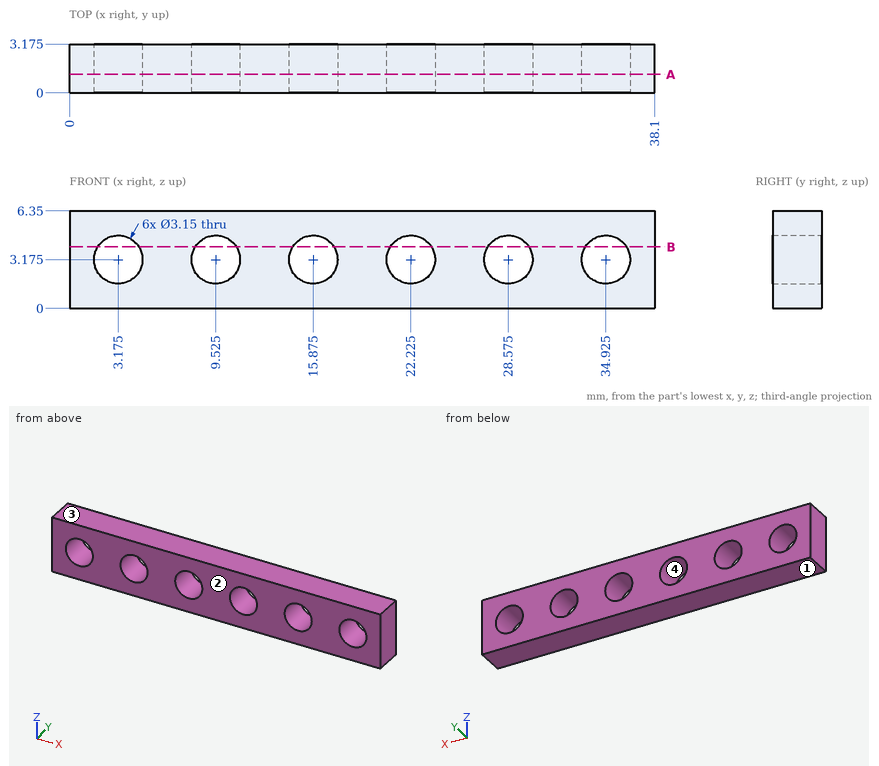
The drawing under review shows one solid part. Ordinate dimensions are in mm from its lowest x, y, z. Round coordinates to 2 decimals unless told otherwise and drop trailing zeros. Write each loop counter-clockwise with the first axis right and the second up, starting at its lowest first coordinate (ties: lowest second). Pieces come first, ordered by that corner, then holes.
(1) Wall thickness on L1, parallel to Z at x = 35, y = 0.95; L2, parallel to Z at x = 2.5, y = 2.3: over which ranges is each line inside the solid? List them lowest first.
(2) We need section A-A on y = 1.2. Give the number of separate pieces and of enclosed holes in the cut face, and give its area (3 significant figures).
(3) We need section B-B on z = 4. Give the boundary of the cut face in (x, y) (1 decimal).
(4) Mouldability with a two-part tool opening along Z and no side actions: class the marked faces 1, 2, 3 and 4 as +Z half, -Z half, draft (parallel to the pull), parting line (faces both ways), or undercut.
Findings below:
1. L1: z = 0 to 1.6, 4.75 to 6.35
1. L2: z = 0 to 1.75, 4.6 to 6.35
2. separate pieces: 1
2. enclosed holes: 6
2. area: 195 mm2
3. outline: (0, 0) - (1.8, 0) - (1.8, 3.2) - (0, 3.2) - close; (4.5, 0) - (8.2, 0) - (8.2, 3.2) - (4.5, 3.2) - close; (10.9, 0) - (14.5, 0) - (14.5, 3.2) - (10.9, 3.2) - close; (17.2, 0) - (20.9, 0) - (20.9, 3.2) - (17.2, 3.2) - close; (23.6, 0) - (27.2, 0) - (27.2, 3.2) - (23.6, 3.2) - close; (29.9, 0) - (33.6, 0) - (33.6, 3.2) - (29.9, 3.2) - close; (36.3, 0) - (38.1, 0) - (38.1, 3.2) - (36.3, 3.2) - close
4. face 1: -Z half
4. face 2: draft
4. face 3: +Z half
4. face 4: undercut
